```python
from build123d import *

# Parameters (mm, degrees)
F0_R     = 480
F0_R_2   = 337.5
F1_DEPTH = 30
F2_R     = 20
F3_DEPTH = 30.001


with BuildPart() as f1:
    # F0 (on Top) → F1 (new body)
    with BuildSketch(Plane.XY):
        Circle(F0_R)
        Circle(F0_R_2, mode=Mode.SUBTRACT)
    extrude(amount=F1_DEPTH)

    # F2 (on face) → F3 (cut, through all)
    with BuildSketch(Plane.XY.offset(30)):
        with Locations((-389.711432, 225)):
            Circle(F2_R)
        with Locations((-450, 0)):
            Circle(F2_R)
        with Locations((-389.711432, -225)):
            Circle(F2_R)
        with Locations((-225, -389.711432)):
            Circle(F2_R)
        with Locations((0, -450)):
            Circle(F2_R)
        with Locations((225, -389.711432)):
            Circle(F2_R)
        with Locations((389.711432, -225)):
            Circle(F2_R)
        with Locations((450, 0)):
            Circle(F2_R)
        with Locations((389.711432, 225)):
            Circle(F2_R)
        with Locations((225, 389.711432)):
            Circle(F2_R)
        with Locations((0, 450)):
            Circle(F2_R)
        with Locations((-225, 389.711432)):
            Circle(F2_R)
    extrude(amount=-F3_DEPTH, mode=Mode.SUBTRACT)


solid = f1.part
```
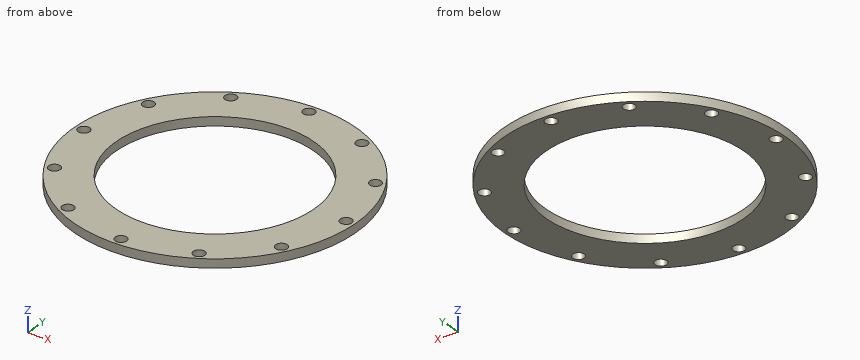
Input: part model. Units: mm. Frame: model coordinates. Round coordinates to 2 decimals unless told otherwise and drop trailing zeros. Loops run counter-clockwise (first coordinate to the right, second up) from the corner with the lowest first, then second, coordinate; pieces in that order, holes last. Notation, with made-up numbers: (16, -20) -> (60, -20) arc R13 cw to (60, -1) -> close; hole circle Ø3 at (28.5, 60.25). An arc over 180 degrees is marked (long way). Use one line per item in the form item = value. Start each with the question number.
Item 1: Material intervals for L1, parallel to Y at x = 0, z = 11.75; L2, parallel to Y at x = -393, z = 12; L3, parallel to X at y = 384.5, z = 26.5, sorted ascending. Write a range as from..to.
Item 2: Section query B-B on x = 225. Return the cut outline in (y, z), then the cut area to 3 significant figures.
Item 3: Section query A-A on y = 0. Return the cut outline in (x, z), then the cut area to 3 significant figures.
Item 4: Section query C-C on x = -450. Return the cut outline in (y, z), then the cut area to 3 significant figures.
Item 5: Contact query for flat-ended pins moving along their axis: pin 1 Ø6 at (x, z) = (-158.5, 24) entering from -Y; pin 2 Ø2 at (y, z) = (-351, 24.5) entering from -X; pin 3 Ø8 at (x, z) = (-226, 18) entering from -Y; pin 4 Ø24 at (x, y) = (0, 450) entering from +Z. Output: stop coordinate, or through.
Item 6: Section query D-D on y = -190. Return the cut outline in (x, z).
Ans:
q1.L1 = -480..-470, -430..-337.5, 337.5..430, 470..480
q1.L2 = -275.59..-244.73, -205.27..205.27, 244.73..275.59
q1.L3 = -287.33..-244.31, -205.69..205.69, 244.31..287.33
q2.outline = (-424, 0) -> (-409.71, 0) -> (-409.71, 30) -> (-424, 30) -> close; (-369.71, 0) -> (-251.56, 0) -> (-251.56, 30) -> (-369.71, 30) -> close; (251.56, 0) -> (369.71, 0) -> (369.71, 30) -> (251.56, 30) -> close; (409.71, 0) -> (424, 0) -> (424, 30) -> (409.71, 30) -> close
q2.area = 7,950 mm^2
q3.outline = (-480, 0) -> (-470, 0) -> (-470, 30) -> (-480, 30) -> close; (-430, 0) -> (-337.5, 0) -> (-337.5, 30) -> (-430, 30) -> close; (337.5, 0) -> (430, 0) -> (430, 30) -> (337.5, 30) -> close; (470, 0) -> (480, 0) -> (480, 30) -> (470, 30) -> close
q3.area = 6,150 mm^2
q4.outline = (-167.03, 0) -> (-20, 0) -> (-20, 30) -> (-167.03, 30) -> close; (20, 0) -> (167.03, 0) -> (167.03, 30) -> (20, 30) -> close
q4.area = 8,820 mm^2
q5.pin_1 = -454.11
q5.pin_2 = -328.48
q5.pin_3 = -425.58
q5.pin_4 = through
q6.outline = (-440.79, 0) -> (-278.94, 0) -> (-278.94, 30) -> (-440.79, 30) -> close; (278.94, 0) -> (440.79, 0) -> (440.79, 30) -> (278.94, 30) -> close
